from build123d import *

# Parameters (mm, degrees)
F0_W     = 92.075
F0_H     = 92.075
F1_DEPTH = 25.4
F2_W     = 165.1
F2_H     = 79.756
F3_DEPTH = 19.05
F4_R     = 22.621875
F5_DEPTH = 25.401
F6_W     = 92.075
F6_H     = 6.1595
F7_DEPTH = 6.35
F8_R     = 5.1562
F9_DEPTH = 92.076


with BuildPart() as f1:
    # F0 (on Right) → F1 (new body)
    with BuildSketch(Plane.YZ):
        Rectangle(F0_W, F0_H)
    extrude(amount=F1_DEPTH)

    # F2 (on face) → F3 (cut)
    with BuildSketch(Plane(origin=(0, 0, 0), x_dir=(0, -1, 0), z_dir=(-1, 0, 0))):
        Rectangle(F2_W, F2_H)
    extrude(amount=-F3_DEPTH, mode=Mode.SUBTRACT)

    # F4 (on face) → F5 (cut, through all)
    with BuildSketch(Plane.YZ.offset(25.4)):
        Circle(F4_R)
    extrude(amount=-F5_DEPTH, mode=Mode.SUBTRACT)

    # F6 (on face) → F7 (join)
    with BuildSketch(Plane(origin=(0, 0, 0), x_dir=(0, -1, 0), z_dir=(-1, 0, 0))):
        with Locations((0, 42.95775)):
            Rectangle(F6_W, F6_H)
        with Locations((0, -42.95775)):
            Rectangle(F6_W, F6_H)
    extrude(amount=F7_DEPTH)

    # F8 (on face) → F9 (cut, through all)
    with BuildSketch(Plane.XY.offset(46.0375)):
        with Locations((3.175, -33.3375)):
            Circle(F8_R)
        with Locations((3.175, 33.3375)):
            Circle(F8_R)
    extrude(amount=-F9_DEPTH, mode=Mode.SUBTRACT)


solid = f1.part
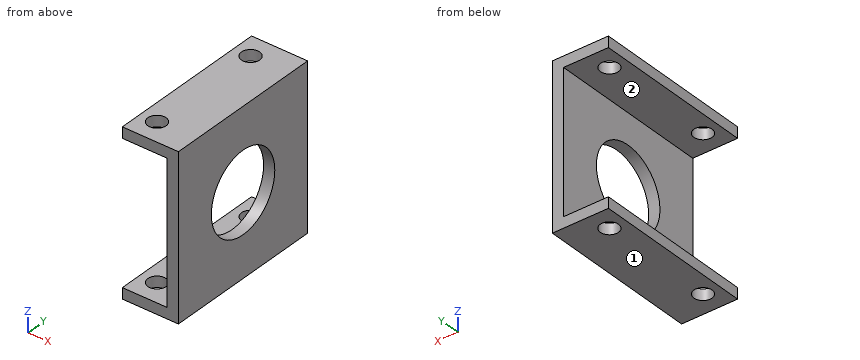
Source: CAD feature listing. Evaluate the final solid. Frame: model axes, mm. Face numbers are marked on the shaded views. A direction names the side the tool comes from. Give positions to 0.01 mm unless a question says otherwise; leave off trailing zeros. Write each loop counter-clockwise with the first axis right and the second up, starting at its lowest first coordinate (ties: lowest second). Pieces come first, ordered by that corner, then holes. Notation, with made-up numbers: (10.5, 17) - (65.5, 17) arc R27 ccw to (65.5, 51) - close; hole circle Ø4 at (-37.75, -38.75). An arc over 180 degrees is marked (long way). Write item = value, one per line. Start each with the question number.
Q1. Material intervals for probe 1 along Z at (x, y) = (21.5, 0); probe 2 along Z at (x, y) = (12, -8); probe 3 along Y at (x, z) = (20, -13.5), sorted ascending.
Q2. Cut plane C-C, the plane x = 14.5. Return loops of the section in (y, z), then the cut area to 3 significant figures.
Q3. Reachability of the marked faces 1 and 2 from +Z, -Z, +X, -X, +Y, -Y: full face, straight path, thin tool, end or side. Return the list, or none.
Q4. Cut plane B-B, the plane z = 0. Return loops of the section in (x, y), then the cut area to 3 significant figures.
Q5. Pin query (flat end, axial travel): pin 1 Ø6 at (x, y) = (3.18, -33.34) entering from +Z. Return the tip coordinate at first contact, or that it passes through.
Q6. Cut plane A-A, the plane y = 0. Return loops of the section in (x, z), then the cut area to 3 significant figures.
Q7. Cut plane D-D, the plane x = 23. Return loops of the section in (y, z), then the cut area to 3 significant figures.
Computed values:
q1.probe_1 = -46.04 to -22.62, 22.62 to 46.04
q1.probe_2 = -46.04 to -39.88, 39.88 to 46.04
q1.probe_3 = -46.04 to -18.15, 18.15 to 46.04
q2.outline = (-46.04, -46.04) - (46.04, -46.04) - (46.04, -39.88) - (-46.04, -39.88) - close; (-46.04, 39.88) - (46.04, 39.88) - (46.04, 46.04) - (-46.04, 46.04) - close
q2.area = 1,130 mm²
q3.face_1 = -Z, +X, -X, +Y, -Y
q3.face_2 = -X, +Y, -Y
q4.outline = (19.05, -46.04) - (25.4, -46.04) - (25.4, -22.62) - (19.05, -22.62) - close; (19.05, 22.62) - (25.4, 22.62) - (25.4, 46.04) - (19.05, 46.04) - close
q4.area = 297 mm²
q5.pin_1 = through
q6.outline = (-6.35, -46.04) - (25.4, -46.04) - (25.4, -22.62) - (19.05, -22.62) - (19.05, -39.88) - (-6.35, -39.88) - close; (-6.35, 39.88) - (19.05, 39.88) - (19.05, 22.62) - (25.4, 22.62) - (25.4, 46.04) - (-6.35, 46.04) - close
q6.area = 610 mm²
q7.outline = (-46.04, -46.04) - (46.04, -46.04) - (46.04, 46.04) - (-46.04, 46.04) - close; hole circle Ø45.24 at (0, 0)
q7.area = 6,870 mm²
